Geometry check sheet. Reference: the model listing, model coordinates, mm. A direction names the side the tool comes from. Coordinates: 2 decimals unless noted, no trailing zeros. Write each loop counter-clockwise with the first axis right and the second up, starting at its lowest first coordinate (ties: lowest second). Pieces come first, ordered by that corner, then holes. Notation, with made-up numbers: (73.25, 56) -> (122.25, 56) arc R21 cw to (122.25, 73) -> close; hole circle Ø6 at (-24.5, 81). An arc over 180 degrees is marked (long way). Answer in a Markdown table with one row per item. Add a question column.
1. Cross-section at D-D on z = -19. Record the cut outline in (x, y), and give its area (3 significant figures).
2. Mould release check, pull along X, two halves, no side actions. Record for faces 6 (the cylindrical face through (30.04, 95.38, -55.86)), 7 (the flat face through (100, 1, -18)), 8 (the cylindrical face through (93.584, -122.297, 4.93)): pulls with the +X half, pulls with the -X half, needs draft (parallel to the pull), parting line crosses it, or undercut.
3. Cross-section at A-A on y = 125. Record the cut outline in (x, z).
4. Cross-section at B-B on z = -53.5. Record the cut outline in (x, y), and give its area (3 significant figures).
5. Cross-section at C-C on x = -85. Give the number of separate pieces and of enclosed holes in the cut face, and give its area (3 significant figures).
6. Set-up check for faces 1 (the flat face through (-100, 1, -18)), 2 (the flat face through (-63, 50, -73)), 3 (the flat face through (-1, -100, -18)), 4 (the flat face through (-68, -46, -36)), 5 (the flat face through (-1, 100, -18)): record each of +Z, -Z, +X, -X, +Y, -Y from which the full face is reachable in a straight line by a thin tool's end or side.
7. Scan lines: L1, parallel to Y at x = 85, z = 4; L2, parallel to Z at x = -90.5, y = 51.5; L3, parallel to X at y = 47, z = -33.5. Record each from-to range of solid material in increasing order. Write a range as from..to.
8. Depth check by flat-ended pin: P1, Ø18, axis at y = -45, z = -24.5, coming from the -X side; P2, Ø2, axis at x = 15, y = 96, coming from the -Z side; P3, Ø1.5, axis at y = 78, z = -68, coming from the +X side. Enter the tip coordinate at first touch or a pass-through.
```python
from build123d import *

# Parameters (mm, degrees)
F0_W     = 220
F0_H     = 300
F0_R     = 9
F1_DEPTH = 10
F2_W     = 200
F2_H     = 200
F3_DEPTH = 36


with BuildPart() as f1:
    # F0 (on Top) → F1 (new body)
    with BuildSketch(Plane.XY):
        Rectangle(F0_W, F0_H)
        with Locations((-85, -125)):
            Circle(F0_R, mode=Mode.SUBTRACT)
        with Locations((85, -125)):
            Circle(F0_R, mode=Mode.SUBTRACT)
        with Locations((-85, 125)):
            Circle(F0_R, mode=Mode.SUBTRACT)
        with Locations((85, 125)):
            Circle(F0_R, mode=Mode.SUBTRACT)
    extrude(amount=F1_DEPTH)

    # F2 (on face) → F3 (join)
    with BuildSketch(Plane(origin=(0, 0, 0), x_dir=(1, 0, 0), z_dir=(0, 0, -1))):
        Rectangle(F2_W, F2_H)
    extrude(amount=F3_DEPTH)

    # F4 (on Right) → F5 (revolve)
    with BuildSketch(Plane.YZ):
        with BuildLine():
            Line((100, -66), (100, -46))
            ThreePointArc((100, -46), (90.250635, -40.725886), (80.224051, -36))
            Line((80.224051, -36), (0, -36))
            Line((0, -36), (0, -83))
            Line((0, -83), (80, -83))
            Line((80, -83), (80, -73))
            Line((80, -73), (95, -73))
            Line((95, -73), (95, -66))
            Line((95, -66), (100, -66))
        make_face()
    revolve(axis=Axis((0, 0, -41.5), (0, 0, -1)))


solid = f1.part
```
Results found:
| question | item | result |
|---|---|---|
| 1 | outline | (-100, -100) -> (100, -100) -> (100, 100) -> (-100, 100) -> close |
| 1 | area | 40,000 mm^2 |
| 2 | face 6 | parting line crosses it |
| 2 | face 7 | pulls with the +X half |
| 2 | face 8 | undercut |
| 3 | outline | (-110, 0) -> (-94, 0) -> (-94, 10) -> (-110, 10) -> close; (-76, 0) -> (76, 0) -> (76, 10) -> (-76, 10) -> close; (94, 0) -> (110, 0) -> (110, 10) -> (94, 10) -> close |
| 4 | outline | circle Ø200 at (0, 0) |
| 4 | area | 31,400 mm^2 |
| 5 | separate pieces | 4 |
| 5 | enclosed holes | 0 |
| 5 | area | 13,100 mm^2 |
| 6 | face 1 | -Z, -X, +Y, -Y |
| 6 | face 2 | -Z |
| 6 | face 3 | -Z, +X, -X, -Y |
| 6 | face 4 | none |
| 6 | face 5 | -Z, +X, -X, +Y |
| 7 | L1 | y = -150..-134, -116..116, 134..150 |
| 7 | L2 | z = -36..10 |
| 7 | L3 | x = -100..100 |
| 8 | P1 | stops at x = -100 |
| 8 | P2 | stops at z = -66 |
| 8 | P3 | stops at x = 55.29 |
